Can you work these out from the model? Positions are in its coordinate system, mm. A direction names the side the tool comes from. Give positions to 0.01 mm unless a question says otherwise; leave off trailing zeros. Write each loop counter-clockwise with the first axis right and the second up, starting at its lowest first coordinate (ties: lowest second). Pieces come first, ordered by that corner, then holes.
Autodesk Inventor part; units mm, degrees
ref_plane "YZ Plane" through (0, 0, 0) normal (1, 0, 0) x (0, 1, 0)
ref_plane "XZ Plane" through (0, 0, 0) normal (0, 1, 0) x (-1, 0, 0)
ref_plane "XY Plane" through (0, 0, 0) normal (0, 0, 1) x (1, 0, 0)
sketch "Sketch1" plane through (0, 0, 0) normal (0, 1, 0) x (-1, 0, 0)
  line L0 (0, 0) -> (0, -42)
  line L1 (0, -42) -> (10, -42)
  line L2 (10, -42) -> (10, 0)
  line L3 (10, 0) -> (0, 0)
  dimension "d0" = 42
  dimension "d1" = 10
  dimension "d2" = 42
extrude "Extrusion1" add sketch "Sketch1" along normal blind 200
sketch "Sketch2" plane through (0, 0, 0) normal (1, 0, 0) x (0, 0, -1)
  line L0 (42, 200) -> (0, 200)
  line L1 (42, 200) -> (42, 161.5)
  line L2 (42, 0) -> (42, 200)
  line L3 (42, 161.5) -> (0, 161.5)
  line L4 (0, 0) -> (0, 200)
  line L5 (0, 161.5) -> (0, 153.5)
  line L6 (0, 153.5) -> (42, 153.5)
  line L7 (42, 153.5) -> (42, 161.5)
  dimension "d5" = 38.5
  dimension "d6" = 8
extrude "Extrusion2" add sketch "Sketch2" along normal blind 10 contours L2 L6 L4 L3
sketch "Sketch3" plane through (-10, 0, -42) normal (-1, 0, 0) x (0, 0, 1)
  line L0 (42, 161.5) -> (42, 200)
  line L1 (42, 200) -> (42, 161.5)
  line L2 (42, 161.5) -> (0, 161.5)
  line L3 (0, 153.5) -> (42, 153.5)
  line L4 (0, 161.5) -> (0, 153.5)
  line L5 (42, 161.5) -> (42, 153.5)
  line L6 (0, 153.5) -> (42, 153.5)
  line L7 (42, 153.5) -> (42, 161.5)
  point P0 (42, 0)
  dimension "d9" = 38.5
extrude "Extrusion3" add sketch "Sketch3" along normal blind 10
sketch "Sketch4" plane through (-10, 0, -42) normal (-1, 0, 0) x (0, 0, 1)
  line L0 (42, 0) -> (42, 153.5)
  line L1 (42, 18.0001) -> (0, 57.4937)
  line L2 (0, 0) -> (0, 153.5)
  circle A0 centre (21, 37.7469) radius 2.65
  dimension "d12" = 5.3
extrude "Extrusion4" cut sketch "Sketch4" against normal blind 10
properties part number "pared"
1) Suppose I cut it at B-B on y = 108. Write out the boundary of the cut face in (x, z).
Values follow:
outline: (-10, -42) - (0, -42) - (0, 0) - (-10, 0) - close
2) Please list where these lines run through material, in increasing order: L1, parallel to Y at x = -5, z = -21; L2, parallel to Y at x = 1.25, z = -11.5; L3, parallel to X at y = 142, z = -23.5.
Values follow:
L1: y = 0 to 35.1, 40.4 to 200
L2: y = 153.5 to 161.5
L3: x = -10 to 0
3) Suppose I cut it at A-A on z = -21. Write out the boundary of the cut face in (x, y).
Values follow:
outline: (-20, 153.5) - (-10, 153.5) - (-10, 40.4) - (0, 40.4) - (0, 153.5) - (10, 153.5) - (10, 161.5) - (0, 161.5) - (0, 200) - (-10, 200) - (-10, 161.5) - (-20, 161.5) - close; (-10, 0) - (0, 0) - (0, 35.1) - (-10, 35.1) - close
4) Suppose I cut it at C-C on x = -17. Write out the boundary of the cut face in (y, z), plus the area to 3 significant figures.
Values follow:
outline: (153.5, -42) - (161.5, -42) - (161.5, 0) - (153.5, 0) - close
area: 336 mm2
5) For pin 1 Ø8 at (x, z) = (-16.5, -18) entering from +Y; pin 2 Ø11.5 at (y, z) = (185.5, -26) entering from -X; pin 3 Ø8 at (y, z) = (138.5, -6.5) entering from +X, each with a flat end and sliding along its axis, tell me the tip position at first contact or that it passes through.
Values follow:
pin 1: stops at y = 161.5
pin 2: stops at x = -10
pin 3: stops at x = 0
6) For faces 1 (the face through (5, 161.5, -21)), 2 (the face through (5, 153.5, -21)), 3 (the face through (-10, 76, -21)), 4 (the face through (-15, 161.5, -21)), which set-ups out of +Z, -Z, +X, -X, +Y, -Y let a thin tool reach every point of the face, with its end or its side?
Values follow:
face 1: +Z, -Z, +X, +Y
face 2: +Z, -Z, +X, -Y
face 3: +Z, -Z, -X, -Y
face 4: +Z, -Z, -X, +Y
7) If we mould it in two halves opening along Y, with no side actions, what happens to faces 5 (the face through (-15, 153.5, -21)), 6 (the face through (0, 76, -21)), 7 (the face through (-5, 200, -21)), 8 (the face through (-5.07, 35.396, -19.777))? For each: +Y half, -Y half, draft (parallel to the pull), parting line (faces both ways), or undercut.
Values follow:
face 5: -Y half
face 6: draft
face 7: +Y half
face 8: undercut
